Autodesk Inventor part; units mm, degrees
ref_plane "YZ Plane" through (0, 0, 0) normal (1, 0, 0) x (0, 1, 0)
ref_plane "XZ Plane" through (0, 0, 0) normal (0, 1, 0) x (-1, 0, 0)
ref_plane "XY Plane" through (0, 0, 0) normal (0, 0, 1) x (1, 0, 0)
sketch "Sketch1" plane through (0, 0, 0) normal (0, 0, 1) x (1, 0, 0)
  circle A0 centre (0, 0) radius 28.75
  line L0 (3.5274, -36.2072) -> (-3.5274, -36.2072)
  line L1 (-3.5274, 36.2072) -> (3.5274, 36.2072)
  arc A1 (3.5274, -36.2072) -> (3.5274, 36.2072) centre (1.7656, 0) ccw
  arc A2 (-3.5274, 36.2072) -> (-3.5274, -36.2072) centre (-1.7656, 0) ccw
  line L2 (3.3345, -28.7072) -> (-3.3345, -28.7072)
  point P0 (0, 0)
  point P1 (0, 36.2072)
  point P2 (0, 0)
  point P3 (0, -28.7072)
  dimension "d0" = 57.5
  dimension "d1" = 36.25
  dimension "d2" = 36.25
  dimension "d8" = 7.0549
extrude "Extrusion1" add sketch "Sketch1" along normal mid plane 10
sketch "Sketch2" plane through (0, 0, 0) normal (0, 0, 1) x (1, 0, 0)
  circle A0 centre (0, 0) radius 28.75
  circle A1 centre (0, 0) radius 18.5625
  dimension "d5" = 37.125
extrude "Extrusion2" add sketch "Sketch2" against normal blind 10
ref_plane "Work Plane1" through (0, 36.2072, 5) normal (-1, 0, 0) x (0, 0, -1)
properties part number "Tilting head - cover side part" material "Steel, Carbon"
Build history of the part. All positions in model axes, mm. A direction names the side the tool comes from. Give positions to 0.01 mm unless a question says otherwise; leave off trailing zeros. Order: outer loops, then holes, each group sorted by start corner. A loop starts at its lowest first (then second) coordinate and runs counter-clockwise, first axis right, second up. Notation, with made-up numbers: M 32.5,38.5 L 90.5,38.5 A23 ccw 90.5,69.5 Z; hole C 25.5,-9.75 d1. An arc over 180 degrees is marked long. Return JSON: item names as keys, results as strings.
Q1. Flat gauge pins, fed straight in: pin 1 (3 mm diameter, centred on x = 13.5, z = -2.5, fed in from -Y); pin 2 (5 mm diameter, centred on y = -21.5, z = -8, fed in from +X); pin 3 (1.5 mm diameter, centred on x = -26.5, y = -7.5, fed in from +Z). Where does each tip first touch, or does it go through?
Answer list:
{"pin 1": "stops at y = -34.78", "pin 2": "stops at x = 21.58", "pin 3": "stops at z = 0"}
Q2. Band-saw the part on C-C (z = 1). Give the cut face in (x, y), then the cut area to 3 significant figures.
Answer list:
{"outline": "M -3.53,-36.21 L 3.53,-36.21 A36.25 ccw 3.53,36.21 L -3.53,36.21 A36.25 ccw Z; hole C 0,0 d57.5", "area": "1,790 mm^2"}
Q3. Two-plate mould, pull along Y, no slides. Class faces 1 (the face through (16, 25, 5)), 2 (the face through (-6.232, 28.066, 2.465)), 3 (the face through (38, 1, 0)), 4 (the face through (-2.416, 18.405, -4.93)): pulls with the +Y half, pulls with the -Y half, needs draft (parallel to the pull), parting line crosses it, or undercut.
Answer list:
{"face 1": "needs draft", "face 2": "undercut", "face 3": "parting line crosses it", "face 4": "undercut"}
Q4. Band-saw the part on D-D (x = 20). Give the cut face in (y, z), then the cut area to 3 significant figures.
Answer list:
{"outline": "M -31.33,-5 L -20.65,-5 L -20.65,-10 L 20.65,-10 L 20.65,-5 L 31.33,-5 L 31.33,5 L 20.65,5 L 20.65,0 L -20.65,0 L -20.65,5 L -31.33,5 Z", "area": "627 mm^2"}
Q5. Band-saw the part on A-A (x = 0). Give the cut face in (y, z), then the cut area to 3 significant figures.
Answer list:
{"outline": "M -36.21,-5 L -28.75,-5 L -28.75,-10 L -18.56,-10 L -18.56,0 L -28.75,0 L -28.75,5 L -36.21,5 Z; M 18.56,-10 L 28.75,-10 L 28.75,-5 L 36.21,-5 L 36.21,5 L 28.75,5 L 28.75,0 L 18.56,0 Z", "area": "353 mm^2"}
Q6. Band-saw the part on B-B (y = 14). Give the cut face in (x, z), then the cut area to 3 significant figures.
Answer list:
{"outline": "M -35.2,-5 L -25.11,-5 L -25.11,-10 L -12.19,-10 L -12.19,0 L -25.11,0 L -25.11,5 L -35.2,5 Z; M 12.19,-10 L 25.11,-10 L 25.11,-5 L 35.2,-5 L 35.2,5 L 25.11,5 L 25.11,0 L 12.19,0 Z", "area": "460 mm^2"}
Q7. Wall check: probe 1 along Y at (x, z) = (0, 3.6); probe 2 along Y at (x, z) = (0, -6); probe 3 along Z at (x, y) = (32.5, -8). Give the ranges that are in metal, low to high. Write a range as from..to.
Answer list:
{"probe 1": "y = -36.21..-28.75, 28.75..36.21", "probe 2": "y = -28.75..-18.56, 18.56..28.75", "probe 3": "z = -5..5"}
Q8. 3-axis set-ups, long thin cutter, end or side, ignore diameter. For faces 5 (the face through (0, -19, -10)), 6 (the face through (16, 25, -5)), 7 (the face through (0, -19, 0)): which of +Z, -Z, +X, -X, +Y, -Y reach the whole face in a straight line?
Answer list:
{"face 5": "-Z, +X, -X, +Y, -Y", "face 6": "-Z", "face 7": "+Z"}
